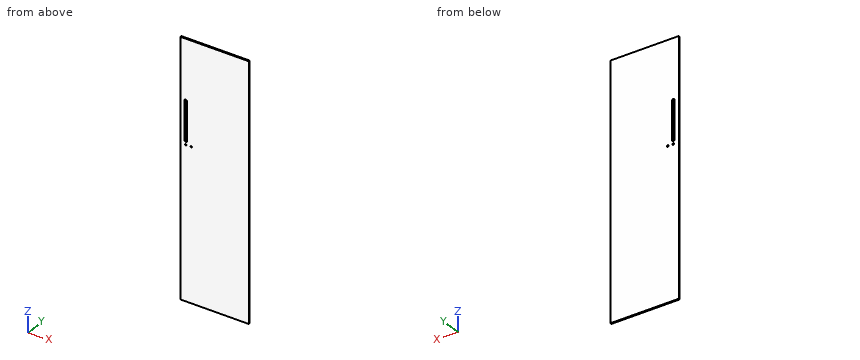
from build123d import *

# Parameters (mm, degrees)
SKETCH1_W                 = 158.75
SKETCH1_H                 = 593.725
BOSS_EXTRUDE1_DEPTH       = 3.175
F_6_CLEARANCE_HOLE1_D     = 3.7973
F_6_CLEARANCE_HOLE1_DEPTH = 12.7
F_6_CLEARANCE_HOLE1_TIP   = 1.140824014
CUT_EXTRUDE3_DEPTH        = 308.307362678


with BuildPart() as part:
    # Sketch1 → Boss-Extrude1 (new body)
    with BuildSketch(Plane(origin=(0, 0, 0), x_dir=(1, 0, 0), z_dir=(0, 1, 0))):
        Rectangle(SKETCH1_W, SKETCH1_H)
    extrude(amount=BOSS_EXTRUDE1_DEPTH)

    # #6 Clearance Hole1
    with Locations(Plane(origin=(0, 3.175, 0), x_dir=(1, 0, 0), z_dir=(0, 1, 0))):
        with Locations((-66.675, -57.099200009), (-53.975, -57.099200009)):
            Hole(F_6_CLEARANCE_HOLE1_D / 2, depth=F_6_CLEARANCE_HOLE1_DEPTH)
            with Locations((0, 0, -(F_6_CLEARANCE_HOLE1_DEPTH + F_6_CLEARANCE_HOLE1_TIP / 2))):  # 118° drill point
                Cone(0, F_6_CLEARANCE_HOLE1_D / 2, F_6_CLEARANCE_HOLE1_TIP, mode=Mode.SUBTRACT)

    # Sketch15 → Cut-Extrude3 (cut, through all)
    with BuildSketch(Plane(origin=(0, 3.175, 0), x_dir=(1, 0, 0), z_dir=(0, 1, 0))):
        with BuildLine():
            Line((-63.4111, -66.941700009), (-63.4111, -155.841700009))
            ThreePointArc((-63.4111, -155.841700009), (-66.675, -159.105600009), (-69.9389, -155.841700009))
            Line((-69.9389, -155.841700009), (-69.9389, -66.941700009))
            ThreePointArc((-69.9389, -66.941700009), (-66.675, -63.677800009), (-63.4111, -66.941700009))
        make_face()
    extrude(amount=-CUT_EXTRUDE3_DEPTH, mode=Mode.SUBTRACT)


solid = part.part
Verification items for the finished model (mm, model axes). Coordinates: 2 decimals unless noted, no trailing zeros. Write each loop counter-clockwise with the first axis right and the second up, starting at its lowest first coordinate (ties: lowest second). Pieces come first, ordered by that corner, then holes. Notation, with made-up numbers: (78, 13.25) - (117, 13.25) arc R14 cw to (117, 34.25) - close; hole circle Ø8 at (-26.5, 67). An arc over 180 degrees is marked (long way). Answer as a JSON object with one key per item and string values.
(1) Gauge pin test, flat end, axial feed: pin 1 Ø2.5 at (x, z) = (-53.98, 57.1) entering from +Y. Record the tip position at first contact, or that the pin passes through.
Report:
{"pin 1": "through"}
(2) Thickness scan on line 1 along X through (y, z) = (2.1, 78.5) (3 decimals); line 2 along Z through (x, y) = (-65, 1.25). Record the ranges inside material, lowest first.
Report:
{"line 1": "-79.375 to -69.939, -63.411 to 79.375", "line 2": "-296.86 to 56.21, 57.99 to 64.14, 158.64 to 296.86"}
(3) Cross-section at A-A on z = 104.5. Record the cut outline in (x, y) (3 decimals), plus the area to 3 significant figures.
Report:
{"outline": "(-79.375, 0) - (-69.939, 0) - (-69.939, 3.175) - (-79.375, 3.175) - close; (-63.411, 0) - (79.375, 0) - (79.375, 3.175) - (-63.411, 3.175) - close", "area": "483 mm^2"}
